Geometry: final body of the model. Coordinates: model frame, mm. Face numbers are marked on the shaded views. A direction names the side the tool comes from. Give positions to 0.01 mm unless a question says otherwise; leave off trailing zeros. Write each loop counter-clockwise with the first axis right and the second up, starting at its lowest first coordinate (ties: lowest second). Pieces come first, ordered by that corner, then holes.
from build123d import *

# Parameters (mm, degrees)
PAD_DEPTH   = 25
FILLET_R    = 3
FILLET001_R = 3
FILLET002_R = 5


with BuildPart() as part:
    # Sketch → Pad (new body, symmetric)
    with BuildSketch(Plane.XY):
        Polygon((0, 37.114174), (0, 0), (-39.984188, 0), (-39.984188, 5), (-5, 5), (-5, 37.114174), align=None)
    extrude(amount=PAD_DEPTH, both=True)

    # Fillet
    fillet_edges = [part.edges().sort_by_distance(p)[0] for p in [
        (-39.984188, 5, 0),
    ]]
    fillet(fillet_edges, radius=FILLET_R)

    # Fillet001
    fillet001_edges = [part.edges().sort_by_distance(p)[0] for p in [
        (-5, 37.114174, 0),
    ]]
    fillet(fillet001_edges, radius=FILLET001_R)

    # Fillet002
    fillet002_edges = [part.edges().sort_by_distance(p)[0] for p in [
        (-5, 5, 0),
    ]]
    fillet(fillet002_edges, radius=FILLET002_R)


solid = part.part
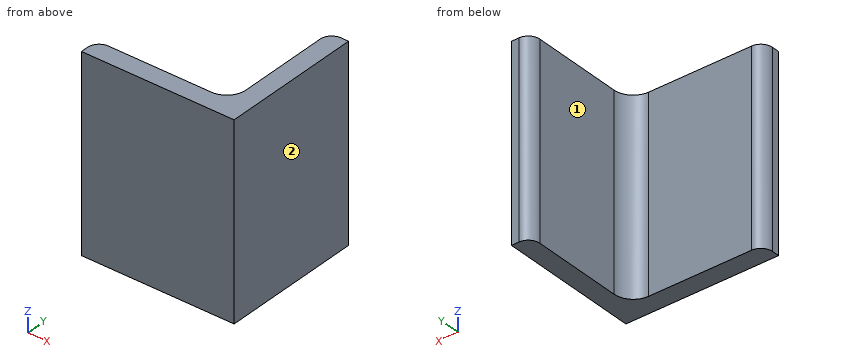
Q1. Ray query, line 1 along X through (y, z) = (20, 20.5); line 2 along Y through (x, z) = (-29, -10); line 3 along Y through (x, z) = (-8, 20.5). Return the intervals inside material, ascending.
Filled sheet:
line 1: x = -5 to 0
line 2: y = 0 to 5
line 3: y = 0 to 5.42
Q2. Section A-A on z = 3.5. Output: boundary loops of the cut face in (x, y), plus the area to 3 significant figures.
Filled sheet:
outline: (-39.98, 0) - (0, 0) - (0, 37.11) - (-2, 37.11) arc R3 ccw to (-5, 34.11) - (-5, 10) arc R5 cw to (-10, 5) - (-36.98, 5) arc R3 ccw to (-39.98, 2) - close
area: 362 mm2
Q3. Section C-C on x = -11. Output: boundary loops of the cut face in (y, z).
Filled sheet:
outline: (0, -25) - (5, -25) - (5, 25) - (0, 25) - close
Q4. Access query for the marked faces 1 and 2. Directions: +Z, -Z, +X, -X, +Y, -Y. A direction counts if a zero-diameter tool reaches every point of the face in a straight line with its end or side. Return the directions, or none.
Filled sheet:
face 1: +Z, -Z, -X, +Y
face 2: +Z, -Z, +X, +Y, -Y
Q5. Pin query (flat end, axial travel): P1, Ø4, axis at y = 14, z = -13.5, coming from the -X side; P2, Ø2, axis at x = -10.5, z = -13.5, coming from the +Y side. Return the tip coordinate at first contact, or that it passes through.
Filled sheet:
P1: stops at x = -5
P2: stops at y = 5.03
Q6. Section B-B on y = 6. Output: boundary loops of the cut face in (x, z).
Filled sheet:
outline: (-7, -25) - (0, -25) - (0, 25) - (-7, 25) - close
